Input: dimensioned drawing with shaded views. Units: mm. Origin: part minimum x, y, z. Round coordinates to 2 decimals unless told otherwise and drop trailing zeros. Loops run counter-clockwise (first coordinate to the right, second up) from the corner with the lowest first, then second, coordinate; pieces in that order, holes last. Notation, with made-up numbers: M 79.5,-4.75 L 115.5,-4.75 A31 ccw 115.5,23.25 Z; hole C -29,75 d5. An arc over 180 degrees is marked long. Return JSON: item names as keys, results as strings.
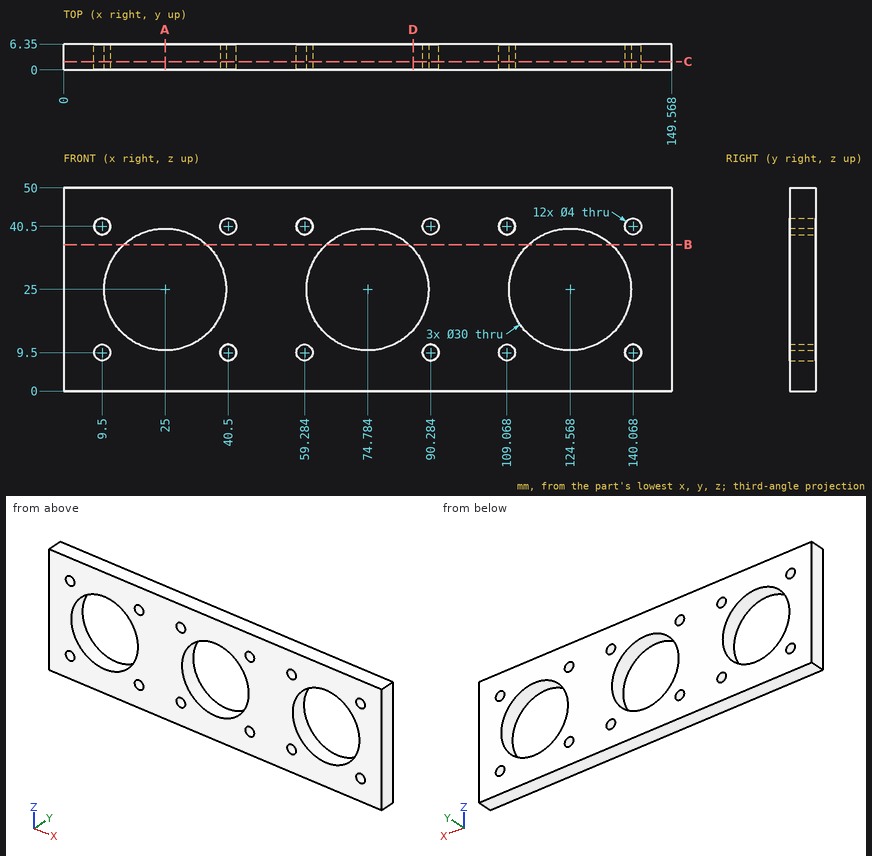
Q1. Material intervals for L1, parallel to X at y = 3.5, z = 25; L2, parallel to X at y = 0.75, z = 18; L3, parallel to Z at x = 141, y = 1.5, sorted ascending.
Determined:
{"L1": "x = 0 to 10, 40 to 59.78, 89.78 to 109.57, 139.57 to 149.57", "L2": "x = 0 to 11.73, 38.27 to 61.52, 88.05 to 111.3, 137.83 to 149.57", "L3": "z = 0 to 7.73, 11.27 to 38.73, 42.27 to 50"}
Q2. Section query A-A (x = 25). Output: boundary loops of the cut face in (y, z), plus the area to 3 significant figures.
Determined:
{"outline": "M 0,0 L 6.35,0 L 6.35,10 L 0,10 Z; M 0,40 L 6.35,40 L 6.35,50 L 0,50 Z", "area": "127 mm^2"}
Q3. Section query B-B (z = 36). Output: boundary loops of the cut face in (x, y).
Determined:
{"outline": "M 0,0 L 14.8,0 L 14.8,6.35 L 0,6.35 Z; M 35.2,0 L 64.59,0 L 64.59,6.35 L 35.2,6.35 Z; M 84.98,0 L 114.37,0 L 114.37,6.35 L 84.98,6.35 Z; M 134.77,0 L 149.57,0 L 149.57,6.35 L 134.77,6.35 Z"}
Q4. Section query D-D (x = 86). Output: boundary loops of the cut face in (y, z).
Determined:
{"outline": "M 0,0 L 6.35,0 L 6.35,15.04 L 0,15.04 Z; M 0,34.96 L 6.35,34.96 L 6.35,50 L 0,50 Z"}
Q5. Section query C-C (y = 2). State how many separate pieces and enclosed holes the cut face has, plus the area to 3 significant figures.
Determined:
{"separate pieces": "1", "enclosed holes": "15", "area": "5,210 mm^2"}
